Verification items for the finished model (mm, model axes). A direction names the side the tool comes from. Round coordinates to 2 decimals unless told otherwise and drop trailing zeros. Order: outer loops, then holes, each group sorted by start corner. A loop starts at its lowest first (then second) coordinate and runs counter-clockwise, first axis right, second up. Notation, with made-up numbers: M 68.25,55.5 L 112.25,55.5 A12 ccw 112.25,59.5 Z; hole C 8.25,7.25 d5. An arc over 180 degrees is marked long. One line per item, written item: value. Start each with the question number.
from build123d import *

# Parameters (mm, degrees)
SKETCH1_W      = 670
SKETCH1_H      = 500
SKETCH1_W_2    = 530
SKETCH1_H_2    = 300
EXTRUDE1_DEPTH = 10
CHAMFER1_SIZE2 = 30
CHAMFER1_SIZE  = 10
CHAMFER2_SIZE2 = 10
CHAMFER2_SIZE  = 30
CHAMFER3_SIZE2 = 30
CHAMFER3_SIZE  = 10
CHAMFER4_SIZE2 = 10
CHAMFER4_SIZE  = 30


with BuildPart() as part:
    # Sketch1 → Extrude1 (new body)
    with BuildSketch(Plane.XY):
        with Locations((335, 250)):
            Rectangle(SKETCH1_W, SKETCH1_H)
        with Locations((335, 250)):
            Rectangle(SKETCH1_W_2, SKETCH1_H_2, mode=Mode.SUBTRACT)
    extrude(amount=EXTRUDE1_DEPTH)

    # Chamfer1
    chamfer1_edges = [part.edges().sort_by_distance(p)[0] for p in [
        (335, 400, 10),
    ]]
    chamfer1_side = [part.faces().sort_by_distance(p)[0] for p in [
        (335, 400, 9.8),
    ]]
    chamfer(chamfer1_edges, length=CHAMFER1_SIZE - 0.0001, length2=CHAMFER1_SIZE2 - 0.0001, reference=chamfer1_side[0])  # a hair under: the kernel refuses the full size

    # Chamfer2
    chamfer2_edges = [part.edges().sort_by_distance(p)[0] for p in [
        (70, 264.99995, 10),
    ]]
    chamfer2_side = [part.faces().sort_by_distance(p)[0] for p in [
        (69.8, 264.99995, 10),
    ]]
    chamfer(chamfer2_edges, length=CHAMFER2_SIZE - 0.0001, length2=CHAMFER2_SIZE2 - 0.0001, reference=chamfer2_side[0])  # a hair under: the kernel refuses the full size

    # Chamfer3
    chamfer3_edges = [part.edges().sort_by_distance(p)[0] for p in [
        (320.00005, 100, 10),
    ]]
    chamfer3_side = [part.faces().sort_by_distance(p)[0] for p in [
        (320.00005, 100, 9.8),
    ]]
    chamfer(chamfer3_edges, length=CHAMFER3_SIZE - 0.0001, length2=CHAMFER3_SIZE2 - 0.0001, reference=chamfer3_side[0])  # a hair under: the kernel refuses the full size

    # Chamfer4
    chamfer4_edges = [part.edges().sort_by_distance(p)[0] for p in [
        (600, 250, 10),
    ]]
    chamfer4_side = [part.faces().sort_by_distance(p)[0] for p in [
        (600.2, 250, 10),
    ]]
    chamfer(chamfer4_edges, length=CHAMFER4_SIZE - 0.0001, length2=CHAMFER4_SIZE2 - 0.0001, reference=chamfer4_side[0])  # a hair under: the kernel refuses the full size


solid = part.part
1. Tool access check on faces 1 (the face through (339, 85, 5)), 2 (the face through (309, 66, 10)). Record the directions out of +Z, -Z, +X, -X, +Y, -Y that give a thin tool (end or side, any length) a straight path to the whole face; none if there is none.
2. Section check C-C (z = 7). Record the cut outline in (x, y), and give its area (3 significant figures).
3. Section check D-D (y = 83.5). Record the cut outline in (x, z), and give its area (3 significant figures).
4. Draft check along X on faces 3 (the face through (330, 420, 0)), 4 (the face through (615, 253, 5)). Enter one of: released by +X, released by -X, zero draft, split by the parting line, or undercut.
5. Scan lines: line 1 along Z through (x, y) = (45, 365); line 2 along Z through (x, y) = (625.5, 379). Record each from-to range of solid material in increasing order.
Geometry check:
1. face 1: +Z
1. face 2: +Z, +X, -X, +Y, -Y
2. outline: M 0,0 L 670,0 L 670,500 L 0,500 Z; hole M 49,79 L 621,79 L 621,421 L 49,421 Z
2. area: 139,000 mm²
3. outline: M 0,0 L 670,0 L 670,10 L 630,10 L 616.5,5.5 L 53.5,5.5 L 40,10 L 0,10 Z
3. area: 4,110 mm²
4. face 3: zero draft
4. face 4: undercut
5. line 1: z = 0 to 8.33
5. line 2: z = 0 to 8.5
